```python
from build123d import *

# Parameters (mm, degrees)
SKETCH1_R           = 16.5
BOSS_EXTRUDE1_DEPTH = 22
SKETCH2_R           = 18.5
BOSS_EXTRUDE2_DEPTH = 19
SKETCH3_R           = 6
BOSS_EXTRUDE3_DEPTH = 6
SKETCH4_R           = 3
BOSS_EXTRUDE4_DEPTH = 15.5
CUT_EXTRUDE1_DEPTH  = 12
SKETCH6_R           = 1.5
CUT_EXTRUDE2_DEPTH  = 5
BOSS_EXTRUDE5_START = 4
SKETCH7_R           = 13
BOSS_EXTRUDE5_DEPTH = 7.5
SKETCH8_W           = 2
SKETCH8_H           = 5
BOSS_EXTRUDE6_DEPTH = 4


with BuildPart() as part:
    # Sketch1 → Boss-Extrude1 (new body)
    with BuildSketch(Plane.XY):
        Circle(SKETCH1_R)
    extrude(amount=BOSS_EXTRUDE1_DEPTH)

    # Sketch2 → Boss-Extrude2 (add)
    with BuildSketch(Plane(origin=(0, 0, 0), x_dir=(-1, 0, 0), z_dir=(0, 0, -1))):
        Circle(SKETCH2_R)
    extrude(amount=BOSS_EXTRUDE2_DEPTH)

    # Sketch3 → Boss-Extrude3 (add)
    with BuildSketch(Plane(origin=(0, 0, -19), x_dir=(-1, 0, 0), z_dir=(0, 0, -1))):
        with Locations((0, 7)):
            Circle(SKETCH3_R)
    extrude(amount=BOSS_EXTRUDE3_DEPTH)

    # Sketch4 → Boss-Extrude4 (add)
    with BuildSketch(Plane(origin=(0, 0, -25), x_dir=(-1, 0, 0), z_dir=(0, 0, -1))):
        with Locations((0, 7)):
            Circle(SKETCH4_R)
    extrude(amount=BOSS_EXTRUDE4_DEPTH)

    # Sketch5 → Cut-Extrude1 (cut)
    with BuildSketch(Plane(origin=(0, 0, -40.5), x_dir=(-1, 0, 0), z_dir=(0, 0, -1))):
        Polygon((-80.661429966, 9.5), (-1.658312395, 9.5), (1.658312395, 9.5), (80.661429966, 9.5), (80.661429966, 167.506235142), (-80.661429966, 167.506235142), align=None)
    extrude(amount=-CUT_EXTRUDE1_DEPTH, mode=Mode.SUBTRACT)

    # Sketch6 → Cut-Extrude2 (cut)
    with BuildSketch(Plane(origin=(0, 0, -19), x_dir=(-1, 0, 0), z_dir=(0, 0, -1))):
        with Locations((-15.5, 0)):
            Circle(SKETCH6_R)
        with Locations((-7.75, 13.423393759)):
            Circle(SKETCH6_R)
        with Locations((7.75, 13.423393759)):
            Circle(SKETCH6_R)
        with Locations((15.5, 0)):
            Circle(SKETCH6_R)
        with Locations((7.75, -13.423393759)):
            Circle(SKETCH6_R)
        with Locations((-7.75, -13.423393759)):
            Circle(SKETCH6_R)
    extrude(amount=-CUT_EXTRUDE2_DEPTH, mode=Mode.SUBTRACT)



with BuildPart() as body_2:
    # Sketch7 → Boss-Extrude5 (new body)
    with BuildSketch(Plane.XY.offset(22).offset(BOSS_EXTRUDE5_START)):
        Circle(SKETCH7_R)
    extrude(amount=BOSS_EXTRUDE5_DEPTH)


with BuildPart() as part_1:
    add(part.part)

    add(body_2.part)  # Boss-Extrude6 merges body 2
    # Sketch8 → Boss-Extrude6 (add)
    with BuildSketch(Plane.XY.offset(22)):
        with Locations((-5.068135622, 0)):
            Rectangle(SKETCH8_W, SKETCH8_H)
        with Locations((5.068135622, 0)):
            Rectangle(SKETCH8_W, SKETCH8_H)
    extrude(amount=BOSS_EXTRUDE6_DEPTH)


solid = part_1.part
```
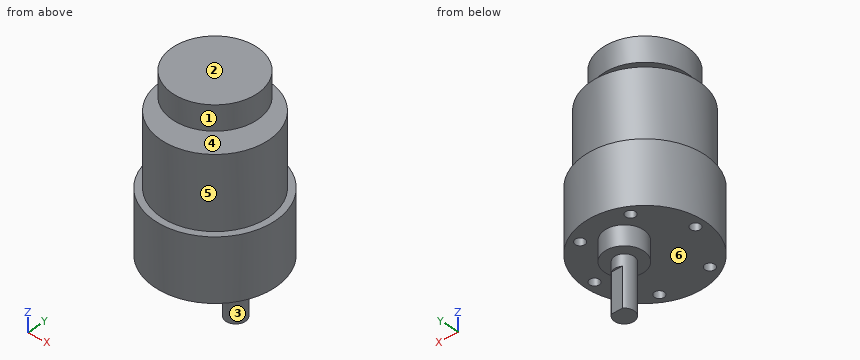
The model under review builds one solid part; all positions refer to its coordinate system, in mm. Face numbers are marked on the shaded views. A direction names the side the tool comes from. Round coordinates to 2 decimals unless told otherwise and drop trailing zeros. Order: outer loops, then holes, each group sorted by start corner. A loop starts at its lowest first (then second) coordinate and runs counter-clockwise, first axis right, second up.
(1) Take a section at B-B, the plane x = 0. State the section outline as (y, z) points, plus the area to 3 significant figures.
Working result:
outline: (-18.5, -19) - (1, -19) - (1, -25) - (4, -25) - (4, -40.5) - (9.5, -40.5) - (9.5, -28.5) - (10, -28.5) - (10, -25) - (13, -25) - (13, -19) - (18.5, -19) - (18.5, 0) - (16.5, 0) - (16.5, 22) - (-16.5, 22) - (-16.5, 0) - (-18.5, 0) - close; (-13, 26) - (13, 26) - (13, 33.5) - (-13, 33.5) - close
area: 1,780 mm2
(2) Take a section at C-C, the plane y = 0. State the section outline as (x, z) points.
Working result:
outline: (-18.5, -19) - (-17, -19) - (-17, -14) - (-14, -14) - (-14, -19) - (14, -19) - (14, -14) - (17, -14) - (17, -19) - (18.5, -19) - (18.5, 0) - (16.5, 0) - (16.5, 22) - (6.07, 22) - (6.07, 26) - (13, 26) - (13, 33.5) - (-13, 33.5) - (-13, 26) - (-6.07, 26) - (-6.07, 22) - (-16.5, 22) - (-16.5, 0) - (-18.5, 0) - close; hole (-4.07, 22) - (4.07, 22) - (4.07, 26) - (-4.07, 26) - close
(3) Mouldability with a two-part tool opening along Z and no side actions: class the marked faces 4, 5 and 6 as released by +Z, released by -Z, zero draft, split by the parting line, or undercut.
Working result:
face 4: undercut
face 5: zero draft
face 6: released by -Z
(4) Take a section at A-A, the plane y = 7. State the section outline as (x, z) points, plus the area to 3 significant figures.
Working result:
outline: (-17.12, -19) - (-6, -19) - (-6, -25) - (-3, -25) - (-3, -40.5) - (3, -40.5) - (3, -25) - (6, -25) - (6, -19) - (17.12, -19) - (17.12, 0) - (14.94, 0) - (14.94, 22) - (-14.94, 22) - (-14.94, 0) - (-17.12, 0) - close; (-10.95, 26) - (10.95, 26) - (10.95, 33.5) - (-10.95, 33.5) - close
area: 1,640 mm2
(5) For P1, Ø1.5, axis at x = -9, y = -3.5, coming from the -Z side; P2, Ø5, axis at x = -8, z = -13, coming from the +Y side; P3, Ø1, axis at x = 4.5, z = 23.5, coming from the +Y side; P4, Ø2, axis at y = 8.5, z = 24.5, coming from the +X side, all flat-tipped, find the tip position at first contact; note any pin that passes through.
Working result:
P1: stops at z = -19
P2: stops at y = 17.66
P3: stops at y = 2.5
P4: passes through
(6) Tool access review of the marked faces 1, 2 and 3: name each direction out of +Z, -Z, +X, -X, +Y, -Y from which nothing blocks a thin tool from reaching the whole face with its end or side.
Working result:
face 1: +Z
face 2: +Z, +X, -X, +Y, -Y
face 3: -Z
(7) Take a section at D-D, the plane z = 2. State the section outline as (x, y) points.
Working result:
outline: circle Ø33 at (0, 0)
(8) Wall thickness on L1, parallel to Z at x = 2, y = 1; L2, parallel to Y at x = 7, z = -15; L3, parallel to Z at x = 3.5, y = 4: over which ranges is each line inside the solid? List them lowest first.
Working result:
L1: z = -19 to 22, 26 to 33.5
L2: y = -17.12 to -14.72, -12.12 to 12.12, 14.72 to 17.12
L3: z = -25 to 22, 26 to 33.5
